```python
from build123d import *

# Parameters (mm, degrees)
ESQUISSE1_R                  = 8
ESQUISSE1_R_2                = 4
BOSS_EXTRU_1_DEPTH           = 2.5
BOSS_EXTRU_2_START           = -2.5
ESQUISSE1_2_R                = 8
ESQUISSE1_2_R_2              = 4
BOSS_EXTRU_2_DEPTH           = 2.5
ENL_V_MAT_EXTRU_1_DEPTH      = 50
ENL_V_MAT_EXTRU_1_DEPTH_BACK = 50
ESQUISSE2_R                  = 1.6


with BuildPart() as part:
    # Esquisse1 → Boss.-Extru.1 (new body)
    with BuildSketch(Plane(origin=(0, 0, 0), x_dir=(1, 0, 0), z_dir=(0, 1, 0))):
        with Locations(Location((0, 0, 0), (0, 0, 270))):
            Circle(ESQUISSE1_R)
        with Locations(Location((0, 0, 0), (0, 0, 270))):
            Circle(ESQUISSE1_R_2, mode=Mode.SUBTRACT)
    extrude(amount=BOSS_EXTRU_1_DEPTH)

    # Esquisse1_2 → Boss.-Extru.2 (add)
    with BuildSketch(Plane(origin=(0, 0, 0), x_dir=(1, 0, 0), z_dir=(0, 1, 0)).offset(BOSS_EXTRU_2_START)):
        with Locations(Location((0, 0, 0), (0, 0, 270))):
            Circle(ESQUISSE1_2_R)
        with Locations(Location((0, 0, 0), (0, 0, 270))):
            Circle(ESQUISSE1_2_R_2, mode=Mode.SUBTRACT)
    extrude(amount=BOSS_EXTRU_2_DEPTH)

    # Esquisse2 → Enl_v. mat.-Extru.1 (cut, two sides: drawn at the far end of the back side and taken through both)
    with BuildSketch(Plane.XY.offset(-ENL_V_MAT_EXTRU_1_DEPTH_BACK)):
        with Locations(Location((0, 0, 0), (0, 0, 180))):
            Circle(ESQUISSE2_R)
    extrude(amount=ENL_V_MAT_EXTRU_1_DEPTH + ENL_V_MAT_EXTRU_1_DEPTH_BACK, mode=Mode.SUBTRACT)


solid = part.part
```
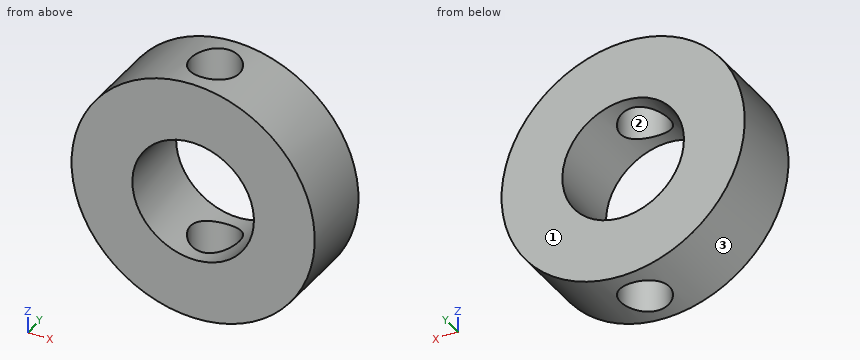
For this review, take the finished solid that the model builds, in its own axes (mm). Face numbers are marked on the shaded views. Round coordinates to 2 decimals unless told otherwise and drop trailing zeros. Write each loop counter-clockwise with the first axis right and the second up, starting at its lowest first coordinate (ties: lowest second). Pieces come first, ordered by that corner, then holes.
1) Take a section at D-D on z = 6.75. Give the boundary of the cut face in (x, y).
Answer below:
outline: (-4.29, -2.5) - (4.29, -2.5) - (4.29, 2.5) - (-4.29, 2.5) - close; hole circle Ø3.2 at (0, 0)
2) Mouldability with a two-part tool opening along X and no side actions: class the marked faces 1, 2 and 3 as +X half, -X half, draft (parallel to the pull), parting line (faces both ways), or undercut.
Answer below:
face 1: draft
face 2: undercut
face 3: parting line
3) Take a section at B-B on y = -0.25. Give the boundary of the cut face in (x, z).
Answer below:
outline: (-1.58, -7.84) - (-1.58, -3.67) arc R4 cw to (-1.58, 3.67) - (-1.58, 7.84) arc R8 ccw to start; (1.58, -7.84) arc R8 ccw to (1.58, 7.84) - (1.58, 3.67) arc R4 cw to (1.58, -3.67) - close
4) Insertion check: pin 1 Ø3 at (x, y) = (-4.5, -1) entering from +Z. The pin has a flat end and moves straight along its axis. Give the tip position at first contact, or say it passes through.
Answer below:
pin 1: stops at z = 7.42
5) For line 1 along X through (y, z) = (0.85, 0); line 2 along Y through (x, z) = (0, 6.1); line 3 along X through (y, z) = (-1.9, 3.5), list the stretches that pass through material, from the lowest coordinate up.
Answer below:
line 1: x = -8 to -4, 4 to 8
line 2: y = -2.5 to -1.6, 1.6 to 2.5
line 3: x = -7.19 to -1.94, 1.94 to 7.19
6) Take a section at C-C on z = -1.25. Give the boundary of the cut face in (x, y).
Answer below:
outline: (-7.9, -2.5) - (-3.8, -2.5) - (-3.8, 2.5) - (-7.9, 2.5) - close; (3.8, -2.5) - (7.9, -2.5) - (7.9, 2.5) - (3.8, 2.5) - close
7) Take a section at A-A on x = 0. Give the boundary of the cut face in (y, z).
Answer below:
outline: (-2.5, -8) - (-1.6, -8) - (-1.6, -4) - (-2.5, -4) - close; (-2.5, 4) - (-1.6, 4) - (-1.6, 8) - (-2.5, 8) - close; (1.6, -8) - (2.5, -8) - (2.5, -4) - (1.6, -4) - close; (1.6, 4) - (2.5, 4) - (2.5, 8) - (1.6, 8) - close
